from build123d import *

# Parameters (mm, degrees)
CROQUIS1_R              = 5.5
CROQUIS1_R_2            = 3.225
SALIENTE_EXTRUIR1_DEPTH = 4.25
CROQUIS3_R              = 4.85
CROQUIS3_R_2            = 2.1
SALIENTE_EXTRUIR2_DEPTH = 3
REDONDEO1_R             = 0.6
CROQUIS4_R              = 3.2
CORTAR_EXTRUIR1_DEPTH   = 1
CORTAR_EXTRUIR2_START   = -0.7
CROQUIS5_W              = 4.1
CROQUIS5_H              = 5
CORTAR_EXTRUIR2_DEPTH   = 12.333085159
REDONDEO2_R             = 1
REDONDEO3_R             = 0.75


with BuildPart() as part:
    # Croquis1 → Saliente-Extruir1 (new body)
    with BuildSketch(Plane(origin=(0, 0, 0), x_dir=(1, 0, 0), z_dir=(0, 1, 0))):
        with Locations(Location((0, 0, 0), (0, 0, 270))):
            Circle(CROQUIS1_R)
        with Locations(Location((0, 0, 0), (0, 0, 270))):
            Circle(CROQUIS1_R_2, mode=Mode.SUBTRACT)
    extrude(amount=SALIENTE_EXTRUIR1_DEPTH)

    # Croquis2 → Revolución1 (revolve)
    with BuildSketch(Plane.XY, mode=Mode.PRIVATE) as revoluci_n1_sk:
        Polygon((-5.5, 4.25), (-4.85, 5.25), (-2.1, 5.25), (-2.1, 5.15), (-3.225, 4.25), align=None)
    revolve(revoluci_n1_sk.sketch.rotate(Axis((0, 0, 0), (0, 1, 0)), 270), axis=Axis((0, 0, 0), (0, 1, 0)))

    # Croquis3 → Saliente-Extruir2 (add)
    with BuildSketch(Plane(origin=(0, 5.25, 0), x_dir=(1, 0, 0), z_dir=(0, 1, 0))):
        with Locations(Location((0, 0, 0), (0, 0, 270))):
            Circle(CROQUIS3_R)
        with Locations(Location((0, 0, 0), (0, 0, 90))):
            Circle(CROQUIS3_R_2, mode=Mode.SUBTRACT)
    extrude(amount=SALIENTE_EXTRUIR2_DEPTH)

    # Redondeo1
    redondeo1_edges = [part.edges().sort_by_distance(p)[0] for p in [
        (0, 8.25, -4.85),
    ]]
    fillet(redondeo1_edges, radius=REDONDEO1_R)

    # Croquis4 → Cortar-Extruir1 (cut)
    with BuildSketch(Plane(origin=(0, 8.25, 0), x_dir=(1, 0, 0), z_dir=(0, 1, 0))):
        with Locations(Location((0, 0, 0), (0, 0, 270))):
            Circle(CROQUIS4_R)
    extrude(amount=-CORTAR_EXTRUIR1_DEPTH, mode=Mode.SUBTRACT)

    # Croquis5 → Cortar-Extruir2 (cut, through all)
    with BuildSketch(Plane(origin=(0, 7.25, 0), x_dir=(1, 0, 0), z_dir=(0, 1, 0)).offset(CORTAR_EXTRUIR2_START)):
        with Locations((0, 2.503070431)):
            Rectangle(CROQUIS5_W, CROQUIS5_H)
    extrude(amount=CORTAR_EXTRUIR2_DEPTH, mode=Mode.SUBTRACT)

    # Redondeo2
    redondeo2_edges = [part.edges().sort_by_distance(p)[0] for p in [
        (0, 5.15, 2.1),
    ]]
    fillet(redondeo2_edges, radius=REDONDEO2_R)

    # Redondeo3
    redondeo3_edges = [part.edges().sort_by_distance(p)[0] for p in [
        (0, 0, -3.225),
    ]]
    fillet(redondeo3_edges, radius=REDONDEO3_R)


solid = part.part
Can you work these out from the model? Positions are in its coordinate system, mm. A direction names the side the tool comes from. Give positions to 0.01 mm unless a question says otherwise; leave off trailing zeros. Loops run counter-clockwise (first coordinate to the right, second up) from the corner with the lowest first, then second, coordinate; pieces in that order, holes last. Notation, with made-up numbers: (-1, -9.75) - (9, -9.75) arc R26 ccw to (9, 27.25) - close; hole circle Ø11 at (-8.5, 49). An arc over 180 degrees is marked (long way). One line per item, written item: value.
(1) On a 3-axis mill with a long thin cutter (end or side, diameter ignored), from which of +Z, -Z, +X, -X, +Y, -Y can I reach the whole of each face in a straight line? I mean faces 1 (the face through (-0.7, 7.25, 2.2)), 2 (the face through (2.05, 7, -3)), 3 (the face through (-3.15, 2.48, -0.7)). Say none if no direction works.
Verdict:
face 1: +Y
face 2: -Z, +Y
face 3: -Y
(2) I'm going to push flat-ended pins straight in: pin 1 (1.5 mm diameter, centred on y = 5.5, z = 1, fed in from +X); pin 2 (2 mm diameter, centred on x = 0, z = -2, fed in from +Y); pin 3 (1.5 mm diameter, centred on x = 2, y = 3, fed in from +Z); pin 4 (6 mm diameter, centred on x = 0, z = 1, fed in from +Y). Where does each tip first touch, or does it pass through?
Verdict:
pin 1: x = 5.1
pin 2: y = 6.55
pin 3: z = 5.36
pin 4: y = 8.25
(3) If we section it at A-A, the plane y = 6.75: List the corners of the cut face in (x, z) for me, plus the area to 3 significant figures.
Verdict:
outline: (-2.05, -4.4) - (-2.05, -0.46) arc R2.1 cw (long way) to (2.05, -0.46) - (2.05, -4.4) arc R4.85 ccw (long way) to start
area: 47.7 mm^2
(4) I need wall thicknesses on line 1 along X through (y, z) = (6.65, 0); line 2 along X through (y, z) = (2.5, -0.75); line 3 along Z through (x, y) = (1, 5.5). Which ranges of each line are inside material? Lowest first, please.
Verdict:
line 1: -4.85 to -2.1, 2.1 to 4.85
line 2: -5.45 to -3.14, 3.14 to 5.45
line 3: -4.75 to -1.86, 1.86 to 4.75
